```python
from build123d import *

# Parameters (mm, degrees)
F1_DEPTH = 330
F3_DEPTH = 30.001
F4_R     = 2.6
F5_DEPTH = 50.001
F6_SIZE  = 2.25


with BuildPart() as f1:
    # F0 (on Front) → F1 (new body)
    with BuildSketch(Plane.XZ):
        with BuildLine():
            Line((0, 5), (0, 0))
            Line((0, 0), (5, 0))
            Line((5, 0), (50, 0))
            Line((50, 0), (50, 2.5))
            ThreePointArc((50, 2.5), (49.267766953, 4.267766953), (47.5, 5))
            Line((47.5, 5), (10, 5))
            ThreePointArc((10, 5), (6.4644660941, 6.4644660941), (5, 10))
            Line((5, 10), (5, 27.5))
            ThreePointArc((5, 27.5), (4.267766953, 29.267766953), (2.5, 30))
            Line((2.5, 30), (0, 30))
            Line((0, 30), (0, 5))
        make_face()
    extrude(amount=-F1_DEPTH)

    # F2 (on face) → F3 (cut, through all)
    with BuildSketch(Plane.XY.offset(30)):
        Polygon((2.5, 330), (2.5, 327.5), (72.6712993005, 257.3287006995), (72.6712993005, 330), align=None)
        Polygon((72.6712993005, 72.6712993005), (2.5, 2.5), (2.5, 0), (72.6712993005, 0), align=None)
        Polygon((2.5, 330), (0, 330), (2.5, 327.5), align=None)
        Polygon((2.5, 2.5), (0, 0), (2.5, 0), align=None)
    extrude(amount=-F3_DEPTH, mode=Mode.SUBTRACT)

    # F4 (on face) → F5 (cut, through all)
    with BuildSketch(Plane(origin=(0, 0, 0), x_dir=(0, -1, 0), z_dir=(-1, 0, 0))):
        with Locations((-85, 17)):
            Circle(F4_R)
        with Locations((-60, 17)):
            Circle(F4_R)
    extrude(amount=-F5_DEPTH, mode=Mode.SUBTRACT)

    # F6
    f6_edges = [f1.edges().sort_by_distance(p)[0] for p in [
        (5, 62.6, 17),
        (5, 87.6, 17),
    ]]
    chamfer(f6_edges, length=F6_SIZE)


solid = f1.part
```
Input: part model. Units: mm. Frame: model coordinates. A direction names the side the tool comes from. Give positions to 0.01 mm unless a question says otherwise; leave off trailing zeros. Write each loop counter-clockwise with the first axis right and the second up, starting at its lowest first coordinate (ties: lowest second). Pieces come first, ordered by that corner, then holes. Notation, with made-up numbers: (31.25, -24) - (69.25, -24) arc R25 ccw to (69.25, 2) - close; hole circle Ø9 at (89.5, 10.5). An arc over 180 degrees is marked (long way). Write item = value, one per line. Start each with the question number.
1. Access query for faces 1 (the conical face through (2.86, 83.54, 19.28)), 2 (the flat face through (5, 163, 19)). Directions: +Z, -Z, +X, -X, +Y, -Y. A direction counts if a zero-diameter tool reaches every point of the face in a straight line with its end or side. Return the directions, or none.
2. Ray query, L1, parallel to Z at x = 0.7, y = 60; L2, parallel to Z at x = 30, y = 118; L3, parallel to X at y = 90.5, z = 28. Return the intervals inside material, ascending.
3. Section query C-C, the plane y = 289.5. Output: boundary loops of the cut face in (x, z).
4. First-contact query: pin 1 Ø14 at (y, z) = (215, 18) entering from +X; pin 2 Ø3 at (y, z) = (231, 7) entering from +X; pin 3 Ø10 at (x, z) = (22, 6) entering from +Y; pin 4 Ø1.5 at (x, y) = (24.5, 219.5) entering from -Z. Flat tips, straight axial feed; report the tip coordinate or a pass-through.
5. Mould query, pull axis Y, two halves, no side actions, for faces 3 (the flat face through (29, 163, 5)), 4 (the cylindrical face through (1.4, 87.6, 17.1)), 5 (the conical face through (2.86, 58.54, 19.28)), 6 (the flat face through (16, 314, 4)). Classes: released by +Y, released by -Y, zero draft, split by the parting line, or undercut.
6. Section query A-A, the plane y = 172.5. Output: boundary loops of the cut face in (x, z), then the cut area to 3 significant figures.
7. Section query B-B, the plane x = 37. Output: boundary loops of the cut face in (y, z).
Check sheet entries:
q1.face_1 = +X
q1.face_2 = +Z, +X, +Y, -Y
q2.L1 = 0 to 14.4, 19.6 to 30
q2.L2 = 0 to 5
q2.L3 = 0 to 4.95
q3.outline = (0, 0) - (40.5, 0) - (40.5, 5) - (10, 5) arc R5 cw to (5, 10) - (5, 27.5) arc R2.5 ccw to (2.5, 30) - (0, 30) - close
q4.pin_1 = 5
q4.pin_2 = 7.82
q4.pin_3 = 312.9
q4.pin_4 = 0
q5.face_3 = zero draft
q5.face_4 = undercut
q5.face_5 = undercut
q5.face_6 = released by +Y
q6.outline = (0, 0) - (50, 0) - (50, 2.5) arc R2.5 ccw to (47.5, 5) - (10, 5) arc R5 cw to (5, 10) - (5, 27.5) arc R2.5 ccw to (2.5, 30) - (0, 30) - close
q6.area = 378 mm2
q7.outline = (37, 0) - (293, 0) - (293, 5) - (37, 5) - close
